```python
from build123d import *

# Parameters (mm, degrees)
SKETCH_1_R          = 7.5
EXTRUDE_1_DEPTH     = 16
SKETCH_2_R          = 14
EXTRUDE_2_DEPTH     = 4
SKETCH_3_R          = 3
SKETCH_3_R_2        = 1.6
CUT_EXTRUDE_1_DEPTH = 26.455844123
SKETCH_4_R          = 1.6
CUT_EXTRUDE_2_DEPTH = 7.5


with BuildPart() as part:
    # ｽｹｯﾁ1 → ﾎﾞｽ - 押し出し1 (new body)
    with BuildSketch(Plane.XY):
        Circle(SKETCH_1_R)
    extrude(amount=-EXTRUDE_1_DEPTH)

    # ｽｹｯﾁ2 → ﾎﾞｽ - 押し出し2 (add)
    with BuildSketch(Plane.XY):
        Circle(SKETCH_2_R)
    extrude(amount=-EXTRUDE_2_DEPTH)

    # ｽｹｯﾁ3 → ｶｯﾄ - 押し出し1 (cut, through all)
    with BuildSketch(Plane.XY):
        Circle(SKETCH_3_R)
        with Locations((10, 0)):
            Circle(SKETCH_3_R_2)
        with Locations((0, -10)):
            Circle(SKETCH_3_R_2)
        with Locations((-10, 0)):
            Circle(SKETCH_3_R_2)
        with Locations((0, 10)):
            Circle(SKETCH_3_R_2)
    extrude(amount=-CUT_EXTRUDE_1_DEPTH, mode=Mode.SUBTRACT)

    # ｽｹｯﾁ4 → ｶｯﾄ - 押し出し2 (cut)
    with BuildSketch(Plane(origin=(0, 7.5, 0), x_dir=(1, 0, 0), z_dir=(0, 1, 0))):
        with Locations(Location((0, 8, 0), (0, 0, 270))):
            Circle(SKETCH_4_R)
    extrude(amount=-CUT_EXTRUDE_2_DEPTH, mode=Mode.SUBTRACT)


solid = part.part
```
Input: part model. Units: mm. Frame: model coordinates. A direction names the side the tool comes from. Coordinates: 2 decimals unless noted, no trailing zeros. Loops run counter-clockwise (first coordinate to the right, second up) from the corner with the lowest first, then second, coordinate; pieces in that order, holes last. Notation, with made-up numbers: (-17, -29) - (5, -29) arc R33 cw to (5, 6) - close; hole circle Ø7 at (-6.75, 40.25). An arc over 180 degrees is marked (long way). Answer in a Markdown table with one row per item.
(1) Material intervals for L1, parallel to Y at x = 0, z = -1.5; L2, parallel to X at y = -0.75, z = -1; L3, parallel to Z at x = 9, y = -10, sorted ascending. Write a range as from..to.
Model answer:
| item | result |
|---|---|
| L1 | y = -14..-11.6, -8.4..-3, 3..8.4, 11.6..14 |
| L2 | x = -13.98..-11.41, -8.59..-2.9, 2.9..8.59, 11.41..13.98 |
| L3 | z = -4..0 |
(2) Cut plane C-C on y = 2. Output: boundary loops of the cut face in (x, z), plus the area to 3 significant figures.
Model answer:
| item | result |
|---|---|
| outline | (-13.86, -4) - (-7.23, -4) - (-7.23, -16) - (-2.24, -16) - (-2.24, 0) - (-13.86, 0) - close; (2.24, -16) - (7.23, -16) - (7.23, -4) - (13.86, -4) - (13.86, 0) - (2.24, 0) - close |
| area | 213 mm² |
(3) Mould query, pull axis Y, two halves, no side actions, for faces 3 (the face through (6, -6, -4)), 4 (the face through (-0.65, -2.93, -7.89)), 5 (the face through (-1.63, -7.32, -9.92)). Classes: pulls with the +Y half, pulls with the -Y half, needs draft (parallel to the pull), parting line crosses it, or undercut.
Model answer:
| item | result |
|---|---|
| face 3 | needs draft |
| face 4 | undercut |
| face 5 | parting line crosses it |
(4) Cut plane D-D on y = -1.25. Output: boundary loops of the cut face in (x, z), plus the area to 3 significant figures.
Model answer:
| item | result |
|---|---|
| outline | (-13.94, -4) - (-11, -4) - (-11, 0) - (-13.94, 0) - close; (-9, -4) - (-7.4, -4) - (-7.4, -16) - (-2.73, -16) - (-2.73, 0) - (-9, 0) - close; (2.73, -16) - (7.4, -16) - (7.4, -4) - (9, -4) - (9, 0) - (2.73, 0) - close; (11, -4) - (13.94, -4) - (13.94, 0) - (11, 0) - close |
| area | 186 mm² |
(5) Cut plane B-B on x = 10. Output: boundary loops of the cut face in (y, z), plus the area to 3 significant figures.
Model answer:
| item | result |
|---|---|
| outline | (-9.8, -4) - (-1.6, -4) - (-1.6, 0) - (-9.8, 0) - close; (1.6, -4) - (9.8, -4) - (9.8, 0) - (1.6, 0) - close |
| area | 65.6 mm² |
(6) Set-up query: faces 1 (the face through (0.07, 5.05, -9.6)), 2 (the face through (-0.35, 8.44, -1.97)). Return all of +Z, -Z, +X, -X, +Y, -Y with unobstructed straight access to the full face (end or side cutting, diameter ignored); none if empty.
Model answer:
| item | result |
|---|---|
| face 1 | +Y |
| face 2 | +Z, -Z |
(7) Pin query (flat end, axial travel): P1, Ø6, axis at y = -3.5, z = -9.5, coming from the +X side; P2, Ø4, axis at x = 0, z = -8, coming from the -Y side; P3, Ø4, axis at y = -10.5, z = -7, coming from the +X side; P4, Ø3.5, axis at x = 0, y = -10, coming from the -Z side. Return the tip coordinate at first contact, or that it passes through.
Model answer:
| item | result |
|---|---|
| P1 | stops at x = 7.48 |
| P2 | stops at y = -7.5 |
| P3 | passes through |
| P4 | stops at z = -4 |
(8) Cut plane A-A on z = -3. Output: boundary loops of the cut face in (x, y), plus the area to 3 significant figures.
Model answer:
| item | result |
|---|---|
| outline | circle Ø28 at (0, 0); hole circle Ø3.2 at (-10, 0); hole circle Ø6 at (0, 0); hole circle Ø3.2 at (0, -10); hole circle Ø3.2 at (0, 10); hole circle Ø3.2 at (10, 0) |
| area | 555 mm² |
